Check sheet for the modelled part. Datum: model origin and axes. Units: mm. A direction names the side the tool comes from. Round coordinates to 2 decimals unless told otherwise and drop trailing zeros. Loops run counter-clockwise (first coordinate to the right, second up) from the corner with the lowest first, then second, coordinate; pieces in that order, holes last. Notation, with made-up numbers: (17.25, 48.5) -> (23.25, 48.5) arc R34 ccw to (23.25, 78.5) -> close; hole circle Ø7 at (-30.75, -10). An arc over 180 degrees is marked (long way). One line per item, written item: value. Start each with the question number.
1. Cross-section at A-A on x = 0. Record the cut outline in (y, z).
2. Release check for a two-part mould opening along X. For faces 4 (the face through (-3.8, -16, 7.3)), 5 (the face through (-0.2, -14, -8.2)), 6 (the face through (-2.93, -6.9, -13.18)) record: +X half, -X half, draft (parallel to the pull), parting line (faces both ways), or undercut.
3. Cross-section at C-C on y = -14.5. Record the cut outline in (x, z).
4. Go/stop test with flat-tipped pins: pin 1 (8 mm diameter, centred on y = -7.5, z = 2, fed in from +X); pin 2 (5 mm diameter, centred on y = -9.5, z = -6.5, fed in from -X); pin 3 (8 mm diameter, centred on x = -9, y = -4.5, fed in from +Z). Record where each tip stops, or that it passes through.
5. Cross-section at B-B on z = 0. Record the cut outline in (x, y).
6. Set-up check for faces 1 (the face through (-0.2, -2, -8.2)), 2 (the face through (-1.73, -0.99, -7.81)), 3 (the face through (-7, -14, -12)): record each of +Z, -Z, +X, -X, +Y, -Y from which the full face is reachable in a straight line by a thin tool's end or side.
7. Material ranges on L1, parallel to Z at x = 0, y = -15.1; L2, parallel to Z at x = 0, y = -1.05; L3, parallel to Y at x = -9.5, z = 6, recorded low to high.
8. Cross-section at D-D on x = 9.5. Record the cut outline in (y, z).
from build123d import *

# Parameters (mm, degrees)
F0_R     = 13.5
F0_R_2   = 8
F1_DEPTH = 14
F2_R     = 12.5
F3_DEPTH = 12
F4_R     = 16
F4_R_2   = 8
F5_DEPTH = 2


with BuildPart() as f1:
    # F0 (on Front) → F1 (new body)
    with BuildSketch(Plane.XZ):
        Circle(F0_R)
        Circle(F0_R_2, mode=Mode.SUBTRACT)
    extrude(amount=F1_DEPTH)

    # F2 (on face) → F3 (cut)
    with BuildSketch(Plane.XZ.offset(14)):
        Circle(F2_R)
    extrude(amount=-F3_DEPTH, mode=Mode.SUBTRACT)

    # F4 (on face) → F5 (join)
    with BuildSketch(Plane.XZ.offset(14)):
        Circle(F4_R)
        Circle(F4_R_2, mode=Mode.SUBTRACT)
    extrude(amount=F5_DEPTH)


solid = f1.part
Taken from the geometry:
1. outline: (-16, -16) -> (-14, -16) -> (-14, -13.5) -> (0, -13.5) -> (0, -8) -> (-2, -8) -> (-2, -12.5) -> (-14, -12.5) -> (-14, -8) -> (-16, -8) -> close; (-16, 8) -> (-14, 8) -> (-14, 12.5) -> (-2, 12.5) -> (-2, 8) -> (0, 8) -> (0, 13.5) -> (-14, 13.5) -> (-14, 16) -> (-16, 16) -> close
2. face 4: draft
2. face 5: undercut
2. face 6: parting line
3. outline: circle Ø32 at (0, 0); hole circle Ø16 at (0, 0)
4. pin 1: stops at x = 13.5
4. pin 2: stops at x = -12.89
4. pin 3: stops at z = 12.54
5. outline: (-16, -16) -> (-8, -16) -> (-8, -14) -> (-12.5, -14) -> (-12.5, -2) -> (-8, -2) -> (-8, 0) -> (-13.5, 0) -> (-13.5, -14) -> (-16, -14) -> close; (8, -16) -> (16, -16) -> (16, -14) -> (13.5, -14) -> (13.5, 0) -> (8, 0) -> (8, -2) -> (12.5, -2) -> (12.5, -14) -> (8, -14) -> close
6. face 1: none
6. face 2: +Y, -Y
6. face 3: +Y
7. L1: z = -16 to -8, 8 to 16
7. L2: z = -13.5 to -8, 8 to 13.5
7. L3: y = -16 to -14, -2 to 0
8. outline: (-16, -12.87) -> (-14, -12.87) -> (-14, -9.59) -> (0, -9.59) -> (0, 9.59) -> (-14, 9.59) -> (-14, 12.87) -> (-16, 12.87) -> close; hole (-14, -8.12) -> (-2, -8.12) -> (-2, 8.12) -> (-14, 8.12) -> close
